```python
from build123d import *

# Parameters (mm, degrees)
SKETCH1_W               = 7.5
SKETCH1_H               = 5
BOSS_EXTRUDE1_DEPTH     = 10
SKETCH2_R               = 5
BOSS_EXTRUDE2_DEPTH     = 10
CUT_EXTRUDE1_REACH      = 15.463
SKETCH3_R               = 2.75
CUT_EXTRUDE2_DEPTH      = 14.462912018
CUT_EXTRUDE2_DEPTH_BACK = 14.462912018
FILLET1_R               = 1
FILLET3_R               = 1
FILLET4_R               = 1
FILLET1_OF_MIRROR1_R    = 1
CUT_EXTRUDE3_DEPTH      = 23.91287854
CUT_EXTRUDE3_DEPTH_BACK = 23.91287854


with BuildPart() as part:
    # Sketch1 → Boss-Extrude1 (new body)
    with BuildSketch(Plane(origin=(0, 0, 0), x_dir=(1, 0, 0), z_dir=(0, 1, 0))):
        with Locations((3.75, 0)):
            Rectangle(SKETCH1_W, SKETCH1_H)
    boss_extrude1 = extrude(amount=BOSS_EXTRUDE1_DEPTH)

    # Sketch2 → Boss-Extrude2 (add)
    with BuildSketch(Plane(origin=(0, 0, 0), x_dir=(1, 0, 0), z_dir=(0, 1, 0))):
        Circle(SKETCH2_R)
    boss_extrude2 = extrude(amount=BOSS_EXTRUDE2_DEPTH)

    # Sketch3 → Cut-Extrude1 (cut, up to next)
    with BuildSketch(Plane(origin=(0, 0, 0), x_dir=(1, 0, 0), z_dir=(0, 1, 0)), mode=Mode.PRIVATE) as cut_extrude1_sk1:
        with Locations(Location((0, 0, 0), (0, 0, 270))):
            Circle(SKETCH3_R)
    cut_extrude1_tool1 = extrude(cut_extrude1_sk1.sketch, amount=CUT_EXTRUDE1_REACH, mode=Mode.PRIVATE) & part.part
    cut_extrude1 = cut_extrude1_tool1.solids().sort_by_distance((0, 0, 0))[0]
    add(cut_extrude1, mode=Mode.SUBTRACT)

    # Sketch4 → Cut-Extrude2 (cut, two sides: drawn at the far end of the back side and taken through both)
    with BuildSketch(Plane.XY.offset(-CUT_EXTRUDE2_DEPTH_BACK)):
        with BuildLine():
            Line((0, 8), (-5, 8))
            Line((-5, 8), (-5, 2))
            Line((-5, 2), (0, 2))
            Line((0, 2), (4.1, 2))
            ThreePointArc((4.1, 2), (5.35, 5), (4.1, 8))
            Line((4.1, 8), (0, 8))
        make_face()
    extrude(amount=CUT_EXTRUDE2_DEPTH + CUT_EXTRUDE2_DEPTH_BACK, mode=Mode.SUBTRACT)

    # Fillet1
    fillet1_edges = [part.edges().sort_by_distance(p)[0] for p in [
        (4.330127019, 8.876388916, -2.5),
        (4.330127019, 1.123611084, 2.5),
    ]]
    fillet(fillet1_edges, radius=FILLET1_R)

    # Fillet3
    fillet3_edges = [part.edges().sort_by_distance(p)[0] for p in [
        (4.1, 2, 0.002130312),
        (4.1, 8, -0.002130312),
    ]]
    fillet(fillet3_edges, radius=FILLET3_R)

    # Fillet4
    fillet4_edges = [part.edges().sort_by_distance(p)[0] for p in [
        (4.330127019, 1.131174119, -2.5),
        (4.330127019, 8.868825881, 2.5),
    ]]
    fillet(fillet4_edges, radius=FILLET4_R)

    # Mirror1: Boss-Extrude1, Boss-Extrude2, Cut-Extrude1 across plane
    add(boss_extrude1.mirror(Plane(origin=(7.5, 10, -2.5), x_dir=(0, 0, 1), z_dir=(-1, 0, 0))))
    add(boss_extrude2.mirror(Plane(origin=(7.5, 10, -2.5), x_dir=(0, 0, 1), z_dir=(-1, 0, 0))))
    add(cut_extrude1.mirror(Plane(origin=(7.5, 10, -2.5), x_dir=(0, 0, 1), z_dir=(-1, 0, 0))), mode=Mode.SUBTRACT)

    # Fillet1 of Mirror1
    fillet1_of_mirror1_edges = [part.edges().sort_by_distance(p)[0] for p in [
        (10.669872981, 8.876388916, -2.5),
        (10.669872981, 1.123611084, 2.5),
    ]]
    fillet(fillet1_of_mirror1_edges, radius=FILLET1_OF_MIRROR1_R)

    # Sketch6 → Cut-Extrude3 (cut, two sides: drawn at the far end of the back side and taken through both)
    with BuildSketch(Plane.XY.offset(-CUT_EXTRUDE3_DEPTH_BACK)):
        with BuildLine():
            Line((15, 8), (20, 8))
            Line((20, 8), (20, 2))
            Line((20, 2), (15, 2))
            ThreePointArc((15, 2), (12, 5), (15, 8))
        make_face()
    extrude(amount=CUT_EXTRUDE3_DEPTH + CUT_EXTRUDE3_DEPTH_BACK, mode=Mode.SUBTRACT)


solid = part.part
```
Model file for the job. Use its own axes, mm. A direction names the side the tool comes from. Coordinates: 2 decimals unless noted, no trailing zeros. Write each loop counter-clockwise with the first axis right and the second up, starting at its lowest first coordinate (ties: lowest second). Pieces come first, ordered by that corner, then holes. Notation, with made-up numbers: (57.25, -21) - (89.25, -21) arc R29 cw to (89.25, 18) - close; hole circle Ø11 at (-28, -34). An arc over 180 degrees is marked (long way). Use a Markdown table: item, result. Add a question column.
Item 1: Band-saw the part on C-C, the plane x = 0. Write the cut outline in (y, z).
Item 2: Two-plate mould, pull along Z, no slides. Class faces 1 (the face through (4.42, 8.79, 2.61)), 2 (the face through (11.766, 4.93, -3.813)), 3 (the face through (10.589, 4.93, -2.613)), 4 (the face through (-2.685, 0.986, -0.596)): pulls with the +Z half, pulls with the -Z half, needs draft (parallel to the pull), parting line crosses it, or undercut.
Item 3: Band-saw the part on B-B, the plane z = 0. Write the cut outline in (x, y) (3 decimals).
Item 4: Drop flat-ended pins along their axis: pin 1 (1 mm diameter, centred on y = 5, z = -3.5, fed in from -X); pin 2 (3 mm diameter, centred on x = 4, y = 1.5, fed in from +Z); pin 3 (2 mm diameter, centred on x = 10.5, y = 5, fed in from -Z); pin 4 (1.5 mm diameter, centred on x = 1, z = -2.5, fed in from -Y). Give the stop position or say it passes through.
Item 5: Band-saw the part on A-A, the plane y = 1. Write the cut outline in (x, z), and give its area (3 significant figures).
Item 6: 3-axis set-ups, long thin cutter, end or side, ignore diameter. For faces 5 (the face through (8, 5, 2.5)), 6 (the face through (-3, 2, 1)), 7 (the face through (4.411, 1.165, -2.613)), 8 (the face through (18, 8, 0)): which of +Z, -Z, +X, -X, +Y, -Y reach the whole face in a straight line?
Item 7: Drill centre lines: line 1 along X through (y, z) = (8.4, 0); line 2 along Y through (x, z) = (18, -3.5); line 3 along Z through (x, y) = (15, 1.05). Where is each one in solid material? Low to high.
Item 8: Band-saw the part on D-D, the plane z = -3.75. Write the cut outline in (x, y), and give its area (3 significant figures).
A:
| question | item | result |
|---|---|---|
| 1 | outline | (0, -5) - (2, -5) - (2, -2.75) - (0, -2.75) - close; (0, 2.75) - (2, 2.75) - (2, 5) - (0, 5) - close; (8, -5) - (10, -5) - (10, -2.75) - (8, -2.75) - close; (8, 2.75) - (10, 2.75) - (10, 5) - (8, 5) - close |
| 2 | face 1 | pulls with the +Z half |
| 2 | face 2 | parting line crosses it |
| 2 | face 3 | pulls with the -Z half |
| 2 | face 4 | undercut |
| 3 | outline | (-5, 0) - (-2.75, 0) - (-2.75, 2) - (-5, 2) - close; (-5, 8) - (-2.75, 8) - (-2.75, 10) - (-5, 10) - close; (2.75, 0) - (12.25, 0) - (12.25, 3.801) arc R3 cw to (12.25, 6.199) - (12.25, 10) - (2.75, 10) - (2.75, 8) - (3.655, 8) arc R1 cw to (4.439, 7.62) arc R4.225 cw to (4.439, 2.38) arc R1 cw to (3.655, 2) - (2.75, 2) - close; (17.75, 0) - (20, 0) - (20, 2) - (17.75, 2) - close; (17.75, 8) - (20, 8) - (20, 10) - (17.75, 10) - close |
| 4 | pin 1 | stops at x = 11 |
| 4 | pin 2 | stops at z = 4.33 |
| 4 | pin 3 | stops at z = -3.57 |
| 4 | pin 4 | stops at y = 0 |
| 5 | outline | (4.06, -2.92) arc R1 cw to (4.87, -2.5) - (10.13, -2.5) arc R1 cw to (10.94, -2.92) arc R5 ccw (long way) to (10.94, 2.92) arc R1 cw to (10.13, 2.5) - (4.87, 2.5) arc R1 cw to (4.06, 2.92) arc R5 ccw (long way) to start; hole circle Ø5.5 at (0, 0); hole circle Ø5.5 at (15, 0) |
| 5 | area | 137 mm² |
| 6 | face 5 | +Z, +Y, -Y |
| 6 | face 6 | +Z, -Z, -X |
| 6 | face 7 | -Z, +Y, -Y |
| 6 | face 8 | +Z, -Z, +X |
| 7 | line 1 | x = -5 to -2.75, 2.75 to 12.25, 17.75 to 20 |
| 7 | line 2 | y = 0 to 2, 8 to 10 |
| 7 | line 3 | z = -5 to -2.75, 2.75 to 5 |
| 8 | outline | (-3.31, 0) - (3.31, 0) - (3.31, 2) - (-3.31, 2) - close; (-3.31, 8) - (3.31, 8) - (3.31, 10) - (-3.31, 10) - close; (11.69, 0) - (18.31, 0) - (18.31, 2) - (15, 2) arc R3 cw to (15, 8) - (18.31, 8) - (18.31, 10) - (11.69, 10) - close |
| 8 | area | 58.6 mm² |
